The listing builds one solid part. Answer for the finished solid, in the listing's coordinates (mm). A direction names the side the tool comes from. Round coordinates to 2 decimals unless told otherwise and drop trailing zeros. Order: outer loops, then holes, each group sorted by start corner. A loop starts at its lowest first (then second) coordinate and runs counter-clockwise, first axis right, second up. Notation, with made-up numbers: M 74.5,3 L 111.5,3 A17 ccw 111.5,28 Z; hole C 14.25,-2.5 d8. An arc over 180 degrees is marked long. Put each result on its own line as item: value. Start each with the question number.
1. Which of the six approach directions +Z, -Z, +X, -X, +Y, -Y give full straight-line access (tool end or side, diameter ignored) to faces 4 (the face through (37, -10, 2)), 5 (the face through (39, -2.5, 3)), 6 (the face through (43, -4, 5))?
2. The mould has two halves that part along Y. Classify faces 1 (the face through (38, 10, 2)), 2 (the face through (0, 0, 2)), 3 (the face through (17.158, 0, 3)): +Y half, -Y half, draft (parallel to the pull), parting line (faces both ways), or undercut.
3. Each of these flat-tipped pins is pushed along its axis until it touches: pin 1 Ø3 at (x, z) = (67, 1) entering from +Y; pin 2 Ø2.5 at (x, z) = (20, 1.5) entering from -Y. Where does it stop, or does it pass through?
4. The part is cut by section D-D (x = 4). Give the vertices of the cut face in (y, z), then the cut area to 3 significant figures.
5. The part is cut by section C-C (x = 36). Give the vertices of the cut face in (y, z).
6. The part is cut by section B-B (y = 4). Give the vertices of the cut face in (x, z), then the cut area to 3 significant figures.
7. Consider line 1 (Y direction, x = 4, z = 1.1); line 2 (Y direction, x = 59.5, z = 4.15); line 3 (X direction, y = -0.75, z = 3.2). Determine where each line is inside the solid, lowest interval first.
8. The part is cut by section A-A (z = 1.1). Give the vertices of the cut face in (x, y), then the cut area to 3 significant figures.
from build123d import *

# Parameters (mm, degrees)
SCHIZZO1_R                   = 2.5
ESTRUSIONE_ESTRUSIONE1_DEPTH = 5
SCHIZZO2_W                   = 45
SCHIZZO2_H                   = 5
TAGLIO_ESTRUSIONE1_DEPTH     = 89.755250064
SCHIZZO4_R                   = 2
TAGLIO_ESTRUSIONE2_DEPTH     = 89.755250064


with BuildPart() as part:
    # Schizzo1 → Estrusione-Estrusione1 (new body)
    with BuildSketch(Plane.XY):
        with BuildLine():
            Line((0, -10), (75, -10))
            ThreePointArc((75, -10), (88.008053395, 0), (75, 10))
            Line((75, 10), (0, 10))
            Line((0, 10), (0, -10))
        make_face()
        with Locations((77.660254038, 0)):
            Circle(SCHIZZO1_R, mode=Mode.SUBTRACT)
    extrude(amount=ESTRUSIONE_ESTRUSIONE1_DEPTH)

    # Schizzo2 → Taglio-Estrusione1 (cut, through all)
    with BuildSketch(Plane.XY.offset(5)):
        with Locations((39.658388278, 0)):
            Rectangle(SCHIZZO2_W, SCHIZZO2_H)
    extrude(amount=-TAGLIO_ESTRUSIONE1_DEPTH, mode=Mode.SUBTRACT)

    # Schizzo4 → Taglio-Estrusione2 (cut, through all)
    with BuildSketch(Plane.XY.offset(5)):
        with Locations((4, 4)):
            Circle(SCHIZZO4_R)
        with Locations((4, -4)):
            Circle(SCHIZZO4_R)
    extrude(amount=-TAGLIO_ESTRUSIONE2_DEPTH, mode=Mode.SUBTRACT)


solid = part.part
Resolved:
1. face 4: +Z, -Z, -X, -Y
1. face 5: +Z, -Z
1. face 6: +Z, +X, -X, +Y, -Y
2. face 1: +Y half
2. face 2: draft
2. face 3: undercut
3. pin 1: y = 10
3. pin 2: y = -10
4. outline: M -10,0 L -6,0 L -6,5 L -10,5 Z; M -2,0 L 2,0 L 2,5 L -2,5 Z; M 6,0 L 10,0 L 10,5 L 6,5 Z
4. area: 60.0 mm2
5. outline: M -10,0 L -2.5,0 L -2.5,5 L -10,5 Z; M 2.5,0 L 10,0 L 10,5 L 2.5,5 Z
6. outline: M 0,0 L 2,0 L 2,5 L 0,5 Z; M 6,0 L 87.2,0 L 87.2,5 L 6,5 Z
6. area: 416 mm2
7. line 1: -10 to -6, -2 to 2, 6 to 10
7. line 2: -10 to -2.5, 2.5 to 10
7. line 3: 0 to 17.16, 62.16 to 75.28, 80.05 to 87.98
8. outline: M 0,-10 L 75,-10 A10.35 ccw long 75,10 L 0,10 Z; hole C 4,-4 d4; hole C 4,4 d4; hole M 17.16,-2.5 L 62.16,-2.5 L 62.16,2.5 L 17.16,2.5 Z; hole C 77.66,0 d5
8. area: 1,450 mm2
